Verification items for the finished model (mm, model axes). Face numbers are marked on the shaded views. A direction names the side the tool comes from. Coordinates: 2 decimals unless noted, no trailing zeros. Order: outer loops, then holes, each group sorted by start corner. A loop starts at its lowest first (then second) coordinate and runs counter-clockwise, first axis right, second up.
Q1. Cross-section at D-D, the plane y = 47. Record the boundary of the cut face in (x, z).
Q2. Cross-section at B-B, the plane y = -5. Record the boundary of the cut face in (x, z).
Q3. Thickness scan on line 1 (Z direction, x = -5.5, y = 19.5); line 2 (X direction, y = -4.5, z = 10); line 3 (Y direction, x = 10, z = -4.75). Record the ranges inside material, lowest first.
Q4. Depth check by flat-ended pin: P1, Ø6, axis at x = -102.57, y = 79.51, coming from the +Z side; P2, Ø3.5, axis at x = -29.8, y = 81.22, coming from the +Z side; P3, Ø9.5, axis at y = 84, z = -1, coming from the -X side; P4, Ø10.5, axis at x = -39, y = 70.5, coming from the -Z side. Enter the tip coordinate at first touch or a pass-through.
Q5. Set-up check for the marked faces 4, 5 and 6: record each of +Z, -Z, +X, -X, +Y, -Y from which the full face is reachable in a straight line by a thin tool's end or side.
Q6. Cross-section at C-C, the plane x = 10. Record the boundary of the cut face in (y, z).
Q7. Cross-section at A-A, the plane z = -3.5. Record the boundary of the cut face in (x, y) (3 decimals), and give its area (3 significant figures).
Q8. Draft check along X on the marked faces 1, 2 and 3. Enter one of: pulls with the +X half, pulls with the -X half, needs draft (parallel to the pull), parting line crosses it, or undercut.
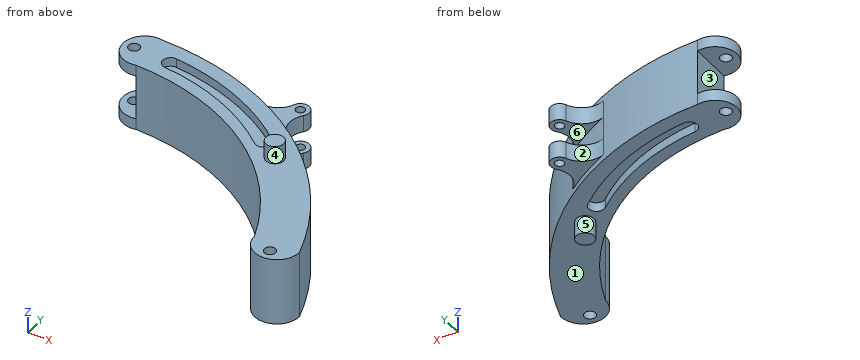
from build123d import *

# Parameters (mm, degrees)
Y_KSEKLIK_EKSTR_ZYON1_DEPTH = 15
Y_KSEKLIK_EKSTR_ZYON2_DEPTH = 5
IZIM4_R                     = 2.5
KES_EKSTR_ZYON1_DEPTH       = 31
Y_KSEKLIK_EKSTR_ZYON3_DEPTH = 12.5
KES_EKSTR_ZYON2_DEPTH       = 5
IZIM7_R                     = 2
KES_EKSTR_ZYON3_DEPTH       = 28.5
IZIM8_R                     = 4
Y_KSEKLIK_EKSTR_ZYON5_DEPTH = 8
KES_EKSTR_ZYON4_DEPTH       = 4
Y_KSEKLIK_EKSTR_ZYON6_DEPTH = 15
IZIM11_R                    = 2.5
KES_EKSTR_ZYON5_DEPTH       = 30


with BuildPart() as part:
    # Çizim1 → Yükseklik-Ekstrüzyon1 (new body, symmetric)
    with BuildSketch(Plane.XY):
        with BuildLine():
            Line((-95.857885087, 89.010731317), (-95.857885087, 70))
            ThreePointArc((-95.857885087, 70), (-37.212348736, 49.675285967), (0, 0))
            Line((0, 0), (20, 0))
            ThreePointArc((20, 0), (-23.570681084, 63.194323514), (-95.857885087, 89.010731317))
        make_face()
    extrude(amount=Y_KSEKLIK_EKSTR_ZYON1_DEPTH, both=True)

    # Çizim3 → Yükseklik-Ekstrüzyon2 (add)
    with BuildSketch(Plane.XY.offset(15)):
        with BuildLine():
            Line((-95.857885087, 89.010731317), (-95.857885087, 70))
            ThreePointArc((-95.857885087, 70), (-107.571379634, 79.505365659), (-95.857885087, 89.010731317))
        make_face()
    y_kseklik_ekstr_zyon2 = extrude(amount=-Y_KSEKLIK_EKSTR_ZYON2_DEPTH)

    # Aynalama1: Yükseklik-Ekstrüzyon2 across plane
    add(y_kseklik_ekstr_zyon2.mirror(Plane.XY))

    # Çizim4 → Kes-Ekstrüzyon1 (cut, through all)
    with BuildSketch(Plane.XY.offset(15)):
        with Locations((-102.571379634, 79.505365659)):
            Circle(IZIM4_R)
    extrude(amount=-KES_EKSTR_ZYON1_DEPTH, mode=Mode.SUBTRACT)

    # Çizim5 → Yükseklik-Ekstrüzyon3 (add, symmetric)
    with BuildSketch(Plane.XY):
        with BuildLine():
            ThreePointArc((-25, 64.276224342), (-35.66270362, 71.406588574), (-47, 77.406676353))
            ThreePointArc((-47, 77.406676353), (-39.114950806, 77.17019229), (-33.511903594, 82.723190348))
            ThreePointArc((-33.511903594, 82.723190348), (-27.753871547, 84.657793137), (-26.723332165, 78.671508013))
            ThreePointArc((-26.723332165, 78.671508013), (-28.951102684, 71.104014108), (-25, 64.276224342))
        make_face()
    extrude(amount=Y_KSEKLIK_EKSTR_ZYON3_DEPTH, both=True)

    # Çizim6 → Kes-Ekstrüzyon2 (cut, symmetric)
    with BuildSketch(Plane.XY):
        with BuildLine():
            ThreePointArc((-25, 64.276224342), (-35.66270362, 71.406588574), (-47, 77.406676353))
            ThreePointArc((-47, 77.406676353), (-39.114950806, 77.17019229), (-33.511903594, 82.723190348))
            ThreePointArc((-33.511903594, 82.723190348), (-27.753871547, 84.657793137), (-26.723332165, 78.671508013))
            ThreePointArc((-26.723332165, 78.671508013), (-28.951102684, 71.104014108), (-25, 64.276224342))
        make_face()
    extrude(amount=KES_EKSTR_ZYON2_DEPTH, both=True, mode=Mode.SUBTRACT)

    # Çizim7 → Kes-Ekstrüzyon3 (cut, through all)
    with BuildSketch(Plane.XY.offset(12.5)):
        with Locations((-29.803865031, 81.223040349)):
            Circle(IZIM7_R)
    extrude(amount=-KES_EKSTR_ZYON3_DEPTH, mode=Mode.SUBTRACT)

    # Çizim8 → Yükseklik-Ekstrüzyon5 (add)
    with BuildSketch(Plane.XY.offset(15)):
        with Locations((-20, 47)):
            Circle(IZIM8_R)
    y_kseklik_ekstr_zyon5 = extrude(amount=Y_KSEKLIK_EKSTR_ZYON5_DEPTH)

    # Aynalama2: Yükseklik-Ekstrüzyon5 across plane
    add(y_kseklik_ekstr_zyon5.mirror(Plane.XY))

    # Çizim9 → Kes-Ekstrüzyon4 (cut)
    with BuildSketch(Plane.XY.offset(15)):
        with BuildLine():
            ThreePointArc((-26.711830739, 56.128041308), (-53.982517061, 73.280029195), (-85.122353286, 81.537850995))
            ThreePointArc((-85.122353286, 81.537850995), (-88.97956649, 78.435931218), (-85.877646714, 74.578718014))
            ThreePointArc((-85.877646714, 74.578718014), (-56.774887256, 66.861098701), (-31.288169261, 50.831143563))
            ThreePointArc((-31.288169261, 50.831143563), (-26.351551127, 51.191423174), (-26.711830739, 56.128041308))
        make_face()
    kes_ekstr_zyon4 = extrude(amount=-KES_EKSTR_ZYON4_DEPTH, mode=Mode.SUBTRACT)

    # Aynalama3: Kes-Ekstrüzyon4 across plane
    add(kes_ekstr_zyon4.mirror(Plane.XY), mode=Mode.SUBTRACT)

    # Çizim10 → Yükseklik-Ekstrüzyon6 (add, symmetric)
    with BuildSketch(Plane.XY):
        with BuildLine():
            Line((0, 0), (20, 0))
            ThreePointArc((20, 0), (10, -10), (0, 0))
        make_face()
    extrude(amount=Y_KSEKLIK_EKSTR_ZYON6_DEPTH, both=True)

    # Çizim11 → Kes-Ekstrüzyon5 (cut)
    with BuildSketch(Plane.XY.offset(15)):
        with Locations((10, -5)):
            Circle(IZIM11_R)
    extrude(amount=-KES_EKSTR_ZYON5_DEPTH, mode=Mode.SUBTRACT)


solid = part.part
Check values:
1. outline: (-33.7, -15) - (-24, -15) - (-24, -23) - (-16, -23) - (-16, -15) - (-6.2, -15) - (-6.2, 15) - (-16, 15) - (-16, 23) - (-24, 23) - (-24, 15) - (-33.7, 15) - close
2. outline: (1.34, -15) - (7.5, -15) - (7.5, 15) - (1.34, 15) - close; (12.5, -15) - (18.66, -15) - (18.66, 15) - (12.5, 15) - close
3. line 1: z = -15 to 15
3. line 2: x = 1.07 to 7.55, 12.45 to 18.93
3. line 3: y = -10 to -7.5, -2.5 to 23.95
4. P1: stops at z = 15
4. P2: passes through
4. P3: stops at x = -95.86
4. P4: stops at z = -15
5. face 4: +Z
5. face 5: -Z
5. face 6: +X, +Y
6. outline: (-10, -15) - (-7.5, -15) - (-7.5, 15) - (-10, 15) - close; (-2.5, -15) - (23.95, -15) - (23.95, 15) - (-2.5, 15) - close
7. outline: (-95.858, 70) arc R106 cw to (0, 0) arc R10 ccw to (20, 0) arc R125 ccw to (-95.858, 89.011) - close; hole circle Ø5 at (10, -5)
7. area: 2,820 mm2
8. face 1: needs draft
8. face 2: undercut
8. face 3: pulls with the -X half
